Autodesk Inventor part; units mm, degrees
ref_plane "YZ Plane" through (0, 0, 0) normal (1, 0, 0) x (0, 1, 0)
ref_plane "XZ Plane" through (0, 0, 0) normal (0, 1, 0) x (-1, 0, 0)
ref_plane "XY Plane" through (0, 0, 0) normal (0, 0, 1) x (1, 0, 0)
sketch "Esquisse1" plane through (0, 0, 0) normal (1, 0, 0) x (0, 1, 0)
  line L0 (0, -56) -> (0, 56)
  line L1 (-49.4, 0) -> (30.4, 0)
  line L2 (-37.5, 32) -> (-37.5, 0)
  line L3 (23.32, 200.2) -> (-20.32, 200.2)
  line L4 (-40.5, 0) -> (-40.5, 32)
  line L5 (-37.5, 0) -> (-40.5, 0)
  line L6 (-40.5, 0) -> (-37.5, 0)
  line L7 (-37.5, 32) -> (-40.5, 32) construction
  line L8 (-37.5, -30) -> (-37.5, 30)
  line L9 (-17.32, -203.2) -> (-17.32, 203.2) construction
  line L10 (-20.32, -203.2) -> (-20.32, 203.2) construction
  line L11 (18.32, 203.2) -> (18.32, -203.2) construction
  line L12 (17.32, -203.2) -> (17.32, 203.2) construction
  line L13 (20.32, -203.2) -> (20.32, 203.2) construction
  line L14 (20.32, 215.2) -> (23.32, 215.2)
  line L15 (23.32, 215.2) -> (23.32, 200.2)
  line L16 (-23.32, 200.2) -> (-23.32, 215.2)
  line L17 (-23.32, 215.2) -> (-20.32, 215.2)
  line L18 (-20.32, 215.2) -> (-20.32, 203.2)
  line L19 (-20.32, 203.2) -> (20.32, 203.2)
  line L20 (20.32, 203.2) -> (20.32, 215.2)
  line L21 (-20.32, 200.2) -> (-23.32, 200.2) construction
  line L22 (20.32, 203.2) -> (20.32, 200.2) construction
  line L23 (-20.32, 200.2) -> (-20.32, 180.2) construction
  line L24 (-20.32, 180.2) -> (-23.32, 170.4614) construction
  line L25 (-23.32, 170.4614) -> (-34.7283, 130.1649) construction
  line L26 (-34.7283, 130.1649) -> (-37.5, 42) construction
  line L27 (-37.5, 42) -> (-37.5, 32) construction
  spline S0 degree 4 poles (-20.32, 200.2) (-20.32, 180.2) (-23.32, 170.4614) (-34.7283, 130.1649) (-37.5, 42) (-37.5, 32) knots 1 1 1 1 1 2 3 3 3 3 3
  spline S1 degree 5 poles (-23.32, 200.2) (-23.32, 198.1335) (-23.3352, 196.0671) (-23.3704, 194.0008) (-23.4817, 190.3714) (-23.7147, 186.748) (-23.8421, 185.1888) (-24.1461, 182.2368) (-24.5662, 179.2992) (-24.7908, 177.914) (-25.3026, 175.0353) (-25.882, 172.1693) (-26.1947, 170.681) (-26.895, 167.4007) (-27.6019, 164.1217) (-27.9836, 162.3284) (-28.8236, 158.3043) (-29.621, 154.2715) (-30.0472, 152.0344) (-30.9633, 147.0388) (-31.8031, 142.0298) (-32.2435, 139.263) (-33.161, 133.1889) (-33.9808, 127.1008) (-34.4002, 123.7858) (-35.2444, 116.7071) (-35.9895, 109.6174) (-36.3603, 105.8482) (-37.0773, 98.0809) (-37.7051, 90.3058) (-38.0066, 86.3042) (-38.5606, 78.4205) (-39.0401, 70.532) (-39.2588, 66.6481) (-39.6316, 59.4781) (-39.9447, 52.3053) (-40.0758, 49.0184) (-40.2667, 43.6432) (-40.4117, 38.2665) (-40.4554, 36.178) (-40.4983, 34.0891) (-40.5, 32) knots 0 0 0 0 0 0 0.060999 0.060999 0.060999 0.107168 0.107168 0.107168 0.148581 0.148581 0.148581 0.193472 0.193472 0.193472 0.247596 0.247596 0.247596 0.314818 0.314818 0.314818 0.397515 0.397515 0.397515 0.496147 0.496147 0.496147 0.607944 0.607944 0.607944 0.726401 0.726401 0.726401 0.841231 0.841231 0.841231 0.938333 0.938333 0.938333 1 1 1 1 1 1
  point P0 (0, 0)
  point P1 (-20.32, 200.2)
  dimension "d9" = 3
  dimension "d16" = 203.2
  dimension "d17" = 12
  dimension "d19" = 32
  dimension "d21" = 20
  dimension "d22" = 10
revolve "Révolution1" add sketch "Esquisse1" angle 360 about axis through (0, -49.4, 0) along (0, 1, 0)
sketch "Esquisse2" plane through (0, 0, 0) normal (0, 1, 0) x (-1, 0, 0)
  circle A0 centre (11, 19.0526) radius 2.5
  circle A1 centre (-11, 19.0526) radius 2.5
  circle A2 centre (-22, 0) radius 2.5
  circle A3 centre (-11, -19.0526) radius 2.5
  circle A4 centre (11, -19.0526) radius 2.5
  circle A5 centre (22, 0) radius 2.5
  circle A6 centre (-11, -19.0526) radius 2.5
  circle A7 centre (11, -19.0526) radius 2.5
  circle A8 centre (22, 0) radius 2.5
  circle A9 centre (11, 19.0526) radius 2.5
  circle A10 centre (-11, 19.0526) radius 2.5
  circle A11 centre (-22, 0) radius 2.5
  circle A12 centre (0, 0) radius 30
  circle A13 centre (0, 0) radius 13
  point P0 (0, 0)
extrude "Extrusion1" cut sketch "Esquisse2" against normal through all contours A0 | A1 | A2 | A3 | A4 | A5
fillet "Congé1" [suppressed]
fillet "Congé3" radius 7.25 1 edges at (0, -20.32, -200.2)
equation "\"d_profile_section\" = 40"
equation "\"d_prfc_thickness\" = 3"
equation "\"d_arm_in_diameter\" = 27"
equation "\"d_arm_out_diameter\" = 30"
equation "\"d_arm_length\" = 250"
equation "\"d_suspension_height\" = 140"
equation "\"d_aluminum_thickness\" = 3.175"
equation "\"d_suspension_box_width\" = 40"
equation "\"d_wheelbase\" = 1600"
equation "\"a_tilt\" = 10deg"
equation "\"d_rear_profile_height\" = 101.6"
equation "\"d_rear_profile_width\" = 50.8"
equation "\"d_central_profile_width\" = 50.8"
equation "\"d_central_profile_height\" = 101.6"
equation "\"d_handle_bar_tube_diameter\" = 35"
equation "\"a_direction_column\" = 35deg"
equation "\"prfc_tube_id\" = 33"
equation "\"prfc_tube_od\" = 35"
equation "\"front_suspension_height\" = 140.92977"
equation "\"front_suspension_width\" = 150"
equation "\"caster_angle\" = 24deg"
equation "\"a_caster_angle\" = 25deg"
equation "\"d_handlebar_pivot_offset\" = 65"
equation "\"d_handlebar_arm_length\" = 80"
equation "\"a_handlebar_angle\" = 60deg"
equation "\"d_left_to_right_front_pivots\" = 28"
equation "\"d_front_arm_id\" = 29.2608"
equation "\"d_front_arm_od\" = 31.75"
equation "\"d_aluminum_bar_thickness\" = 12.7"
equation "\"d_handle_bar_id\" = 30"
equation "\"d_handle_bar_od\" = 38.1"
equation "\"d_steering_arm_length\" = 70"
equation "\"d_steering_height_from_hub_center\" = 28"
equation "\"d_steering_height_from_hub_carrier_center\" = 18"
equation "\"d_central_beam_inclination\" = 12"
equation "\"a_central_beam_inclination\" = 12deg"
equation "\"d_central_beam_screws_diameter\" = 8"
equation "\"d_rear_profile_wall_thickness\" = 4.7625"
equation "\"d_rear_profile_wall_thickness_1\" = 4.7625"
equation "\"d_central_pivot_screw_diameter\" = 15.875"
properties part number "wheel_rim" material "CFRP"
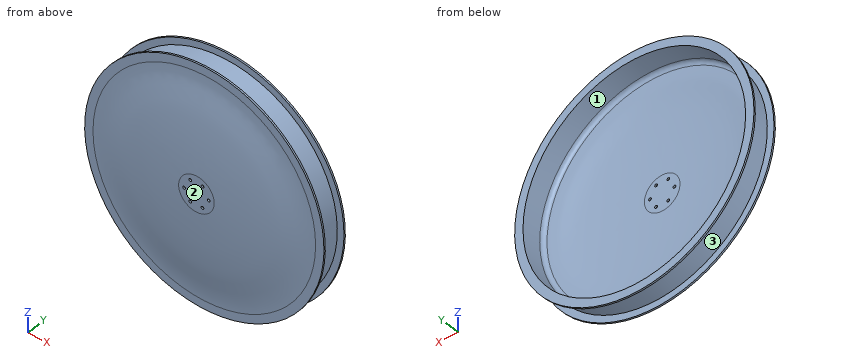
Geometry check sheet. Reference: the model listing, model coordinates, mm. Face numbers are marked on the shaded views. Coordinates: 2 decimals unless noted, no trailing zeros. Order: outer loops, then holes, each group sorted by start corner. A loop starts at its lowest first (then second) coordinate and runs counter-clockwise, first axis right, second up.
Item 1: Depth check by flat-ended pin: pin 1 (1 mm diameter, centred on y = -16, z = -117, fed in from +X); pin 2 (6 mm diameter, centred on x = -142, z = -69, fed in from -Y); pin 3 (1.5 mm diameter, centred on x = 39.5, z = 122, fed in from +Y); pin 4 (3 mm diameter, centred on x = 22, z = 0, fed in from -Y). Enter the tip coordinate at first touch or a pass-through.
Item 2: Section check A-A (y = 4). Enter the section's corners in (x, z), plus the area to 3 significant figures.
Item 3: Scan lines: line 1 along Y through (x, z) = (-79, -190.5); line 2 along Z through (x, y) = (39, 7); line 3 along Y through (x, z) = (-33.5, 0). Record each from-to range of solid material in increasing order.
Item 4: Mould release check, pull along X, two halves, no side actions. Record for the marked faces 1, 2 and 3: released by +X, released by -X, zero draft, split by the parting line, or undercut.
Check sheet entries:
1. pin 1: stops at x = 166.49
1. pin 2: stops at y = -29.49
1. pin 3: stops at y = -30.69
1. pin 4: passes through
2. outline: circle Ø406.4 at (0, 0); hole circle Ø400.4 at (0, 0)
2. area: 3,800 mm2
3. line 1: y = -23.32 to -20.32, 20.32 to 23.32
3. line 2: z = -199.42 to -196.36, 196.36 to 199.42
3. line 3: y = -40.49 to -37.49
4. face 1: undercut
4. face 2: zero draft
4. face 3: split by the parting line
